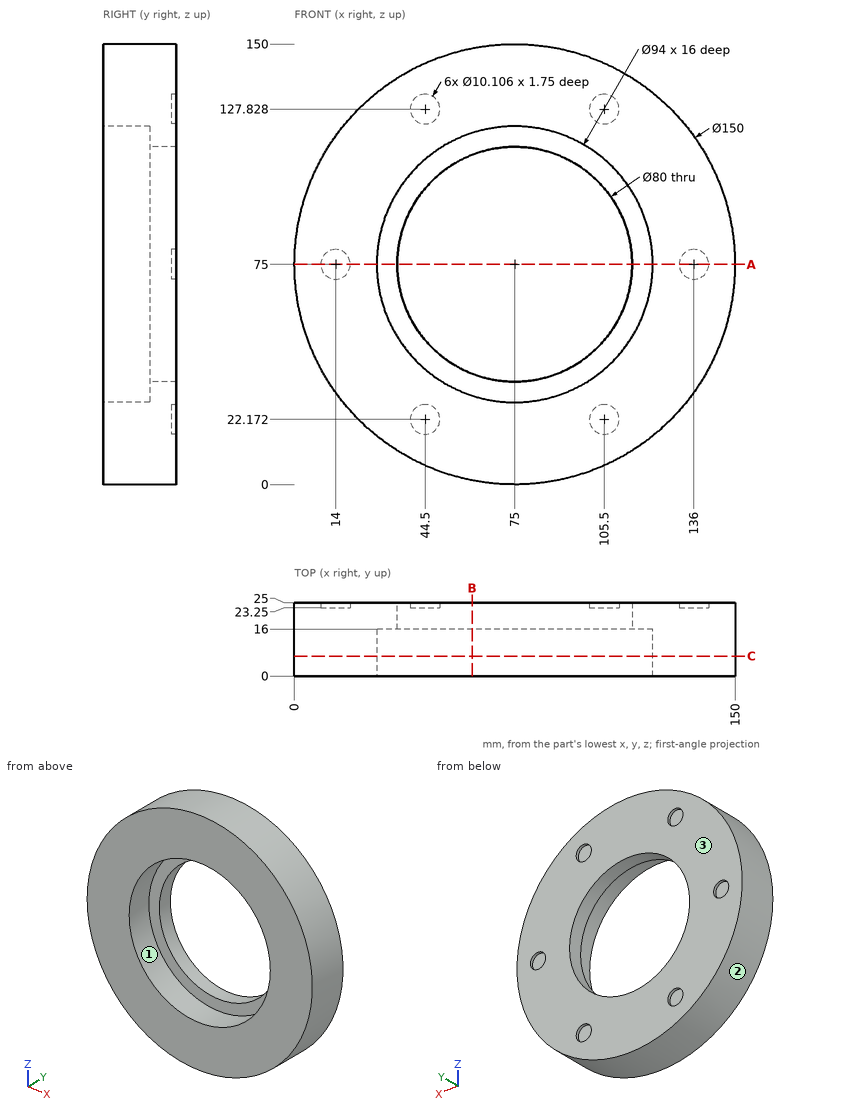
Can you work these out from the drawing? Everything is in mm from the part's minimum corner. Give positions to 0.01 mm unless a question says otherwise; leave off trailing zeros. Order: outer loops, then holes, each group sorted by start corner. A loop starts at its lowest first (then second) coordinate and runs counter-clockwise, first axis right, second up. Notation, with made-up numbers: (-6, 52) -> (1, 52) arc R12 cw to (1, 67) -> close; hole circle Ø11 at (-38, 22). An arc over 180 degrees is marked (long way). Return JSON: item names as keys, results as strings.
1. Thinking about a two-plate mould opening in X: for the marked faces 1, 2 and 3, which applies, pulls with the +X half, pulls with the -X half, needs draft (parallel to the pull), parting line crosses it, or undercut?
Answer list:
{"face 1": "undercut", "face 2": "parting line crosses it", "face 3": "needs draft"}
2. I need wall thicknesses on line 1 (Z direction, x = 105.5, y = 24.15) (1 decimal); line 2 (Z direction, x = 90.5, y = 17.25) (1 decimal); line 3 (Z direction, x = 65, y = 15.5) (1 decimal). Which ranges of each line are inside material? Lowest first, please. Write a range as from..to.
Answer list:
{"line 1": "z = 6.5..17.1, 27.2..49.1, 100.9..122.8, 132.9..143.5", "line 2": "z = 1.6..38.1, 111.9..148.4", "line 3": "z = 0.7..29.1, 120.9..149.3"}
3. Imagine slicing it at B-B on x = 60.5. List the corners of the cut face in (y, z) for me (1 decimal).
Answer list:
{"outline": "(0, 1.4) -> (25, 1.4) -> (25, 37.7) -> (16, 37.7) -> (16, 30.3) -> (0, 30.3) -> close; (0, 119.7) -> (16, 119.7) -> (16, 112.3) -> (25, 112.3) -> (25, 148.6) -> (0, 148.6) -> close"}
4. Imagine slicing it at A-A on z = 75. List the corners of the cut face in (x, y) for me.
Answer list:
{"outline": "(0, 0) -> (28, 0) -> (28, 16) -> (35, 16) -> (35, 25) -> (19.05, 25) -> (19.05, 23.25) -> (8.95, 23.25) -> (8.95, 25) -> (0, 25) -> close; (115, 16) -> (122, 16) -> (122, 0) -> (150, 0) -> (150, 25) -> (141.05, 25) -> (141.05, 23.25) -> (130.95, 23.25) -> (130.95, 25) -> (115, 25) -> close"}
5. For pin 1 Ø8 at (x, z) = (136, 75) entering from +Y; pin 2 Ø4 at (y, z) = (16, 102.5) entering from -X; pin 3 Ø10 at (x, y) = (30, 14) entering from -Z, each with a flat end and sliding along its axis, tell me the tip position at first contact or that it passes through.
Answer list:
{"pin 1": "stops at y = 23.25", "pin 2": "stops at x = 4.47", "pin 3": "stops at z = 11.56"}
6. Imagine slicing it at C-C on y = 6.75. List the corners of the cut face in (x, z) for me.
Answer list:
{"outline": "circle Ø150 at (75, 75); hole circle Ø94 at (75, 75)"}
